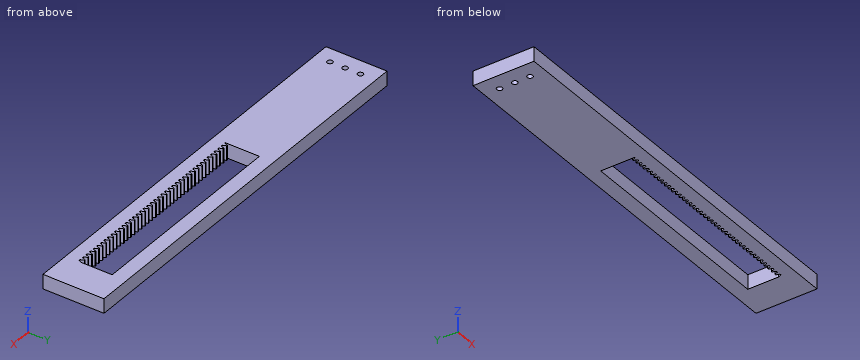
```python
from build123d import *

# Parameters (mm, degrees)
BLANKSKE_W          = 130
BLANKSKE_H          = 10
BLANK_DEPTH         = 9
TOOTHCUTSIM_DEPTH   = 131.694299799
TEETHCUTS_COUNT     = 42
TEETHCUTS_PITCH     = 3.14159265
SKETCH2_W           = 20
SKETCH2_H           = 9
BOSS_EXTRUDE1_DEPTH = 29
SKETCH3_W           = 9
SKETCH3_H           = 9
BOSS_EXTRUDE2_DEPTH = 20
SKETCH3_2_W         = 9
SKETCH3_2_H         = 9
BOSS_EXTRUDE3_DEPTH = 130
SKETCH4_W           = 9
SKETCH4_H           = 38
BOSS_EXTRUDE4_DEPTH = 100
SKETCH5_R           = 1.7
CUT_EXTRUDE1_DEPTH  = 10


with BuildPart() as part:
    # BlankSke → Blank (new body)
    with BuildSketch(Plane.XY):
        with Locations((65, 5)):
            Rectangle(BLANKSKE_W, BLANKSKE_H)
    extrude(amount=-BLANK_DEPTH)

    # TooCutSkeSim → ToothCutSim (cut, through all)
    with BuildSketch(Plane.XY):
        Polygon((0.44443537, 7.75), (-0.44443537, 7.75), (-1.272613241, 10.0254), (1.272613241, 10.0254), align=None)
    toothcutsim = extrude(amount=-TOOTHCUTSIM_DEPTH, mode=Mode.SUBTRACT)

    # TeethCuts: ToothCutSim ×42
    with Locations(*[(i * TEETHCUTS_PITCH, 0, 0) for i in range(1, TEETHCUTS_COUNT)]):
        add(toothcutsim, mode=Mode.SUBTRACT)

    # Sketch2 → Boss-Extrude1 (add)
    with BuildSketch(Plane.XZ):
        with Locations((140, -4.5)):
            Rectangle(SKETCH2_W, SKETCH2_H)
    extrude(amount=-BOSS_EXTRUDE1_DEPTH)

    # Sketch3 → Boss-Extrude2 (add)
    with BuildSketch(Plane.ZY.offset(-130)):
        with Locations((-4.5, 33.5)):
            Rectangle(SKETCH3_W, SKETCH3_H)
    extrude(amount=-BOSS_EXTRUDE2_DEPTH)

    # Sketch3_2 → Boss-Extrude3 (add)
    with BuildSketch(Plane.ZY.offset(-130)):
        with Locations((-4.5, 33.5)):
            Rectangle(SKETCH3_2_W, SKETCH3_2_H)
    extrude(amount=BOSS_EXTRUDE3_DEPTH)

    # Sketch4 → Boss-Extrude4 (add)
    with BuildSketch(Plane.ZY):
        with Locations((-4.5, 19)):
            Rectangle(SKETCH4_W, SKETCH4_H)
    extrude(amount=BOSS_EXTRUDE4_DEPTH)

    # Sketch5 → Cut-Extrude1 (cut)
    with BuildSketch(Plane(origin=(0, 0, -9), x_dir=(-1, 0, 0), z_dir=(0, 0, -1))):
        with Locations((90, 28.5)):
            Circle(SKETCH5_R)
        with Locations((90, 19)):
            Circle(SKETCH5_R)
        with Locations((90, 9.5)):
            Circle(SKETCH5_R)
    extrude(amount=-CUT_EXTRUDE1_DEPTH, mode=Mode.SUBTRACT)


solid = part.part
```
Model file for the job. Use its own axes, mm. Round coordinates to 2 decimals unless told otherwise and drop trailing zeros. Use one line per item in the form item = value.
Item 1: Flat gauge pin, fed straight in: pin 1 Ø4 at (x, y) = (-90, 28.5) entering from -Z. Where does the tip first touch, or does it go through?
Returned:
pin_1 = -9
Item 2: Cut at A-A, the plane z = -6.5. Give the number of separate pieces and of enclosed holes in the cut face, and give its area (3 significant figures).
Returned:
separate_pieces = 1
enclosed_holes = 4
area = 6,840 mm^2
Item 3: Drill centre lines: line 1 (Y direction, x = -90, z = -4.5); line 2 (X direction, y = 20, z = -2); line 3 (X direction, y = 28, z = -6). Where is each one in solid material? Low to high.
Returned:
line_1 = 0 to 7.8, 11.2 to 17.3, 20.7 to 26.8, 30.2 to 38
line_2 = -100 to -91.37, -88.63 to 0, 130 to 150
line_3 = -100 to -91.62, -88.38 to 0, 130 to 150
